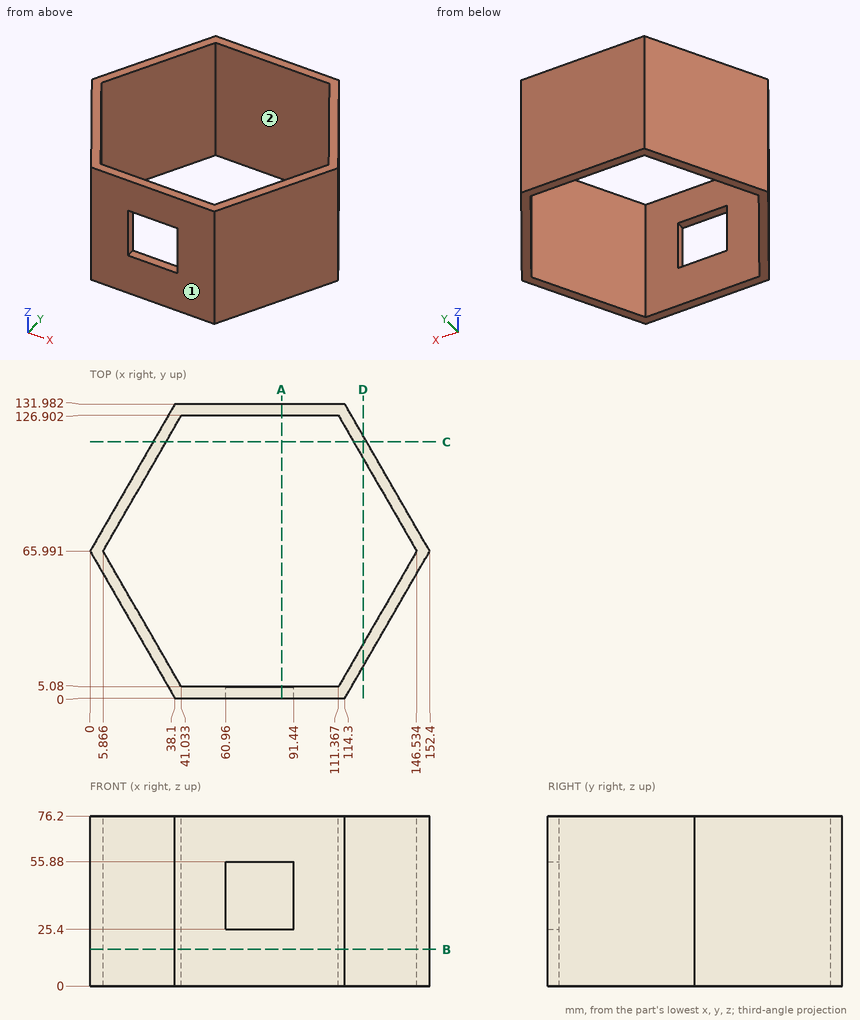
Can you work these out from the drawing? Everything is in mm from the part's minimum corner. A direction names the side the tool comes from. Coordinates: 2 decimals unless noted, no trailing zeros. Loops run counter-clockwise (first coordinate to the right, second up) from the corner with the lowest first, then second, coordinate; pieces in that order, holes last.
1. Imagine slicing it at C-C, the plane y = 115. Please give me the cut outline in (x, z) (1 decimal).
2. Imagine slicing it at A-A, the plane x = 86. Please give me the cut outline in (y, z).
3. For P1, Ø5, axis at x = 119.5, y = 106, coming from the +Z side; P2, Ø3, axis at x = 22, z = 47.5, coming from the +Y side (1 decimal); P3, Ø1.5, axis at y = 1.5, z = 46, coming from the -X side; P4, Ø2, axis at y = 60.5, z = 35, coming from the +X side, each with a flat end and sliding along its axis, tell me the tip position at first contact or that it passes through.
4. Imagine slicing it at D-D, the plane x = 122.5. Please give me the cut outline in (y, z), and give its area (3 significant figures).
5. Imagine slicing it at B-B, the plane z = 16.5. Please give me the cut outline in (x, y).
6. I need wall thicknesses on L1, parallel to Y at x = 87.5, z = 68; L2, parallel to Y at x = 18, z = 45 (1 decimal); L3, parallel to X at y = 5, z = 30. Which ranges of each line are inside material? Lowest first, please.
7. For the marked faces 1 and 2, which set-ups out of +Z, -Z, +X, -X, +Y, -Y let a thin tool reach every point of the face, with its end or its side?
Taken from the geometry:
1. outline: (28.3, 0) - (34.2, 0) - (34.2, 76.2) - (28.3, 76.2) - close; (118.2, 0) - (124.1, 0) - (124.1, 76.2) - (118.2, 76.2) - close
2. outline: (0, 0) - (5.08, 0) - (5.08, 25.4) - (0, 25.4) - close; (0, 55.88) - (5.08, 55.88) - (5.08, 76.2) - (0, 76.2) - close; (126.9, 0) - (131.98, 0) - (131.98, 76.2) - (126.9, 76.2) - close
3. P1: passes through
3. P2: stops at y = 106.7
3. P3: stops at x = 36.8
3. P4: stops at x = 149.81
4. outline: (14.2, 0) - (24.36, 0) - (24.36, 76.2) - (14.2, 76.2) - close; (107.62, 0) - (117.78, 0) - (117.78, 76.2) - (107.62, 76.2) - close
4. area: 1,550 mm2
5. outline: (0, 65.99) - (38.1, 0) - (114.3, 0) - (152.4, 65.99) - (114.3, 131.98) - (38.1, 131.98) - close; hole (5.87, 65.99) - (41.03, 5.08) - (111.37, 5.08) - (146.53, 65.99) - (111.37, 126.9) - (41.03, 126.9) - close
6. L1: y = 0 to 5.08, 126.9 to 131.98
6. L2: y = 34.8 to 45, 87 to 97.2
6. L3: x = 35.21 to 60.96, 91.44 to 117.19
7. face 1: +Z, -Z, +X, -X, -Y
7. face 2: +Z, -Z
